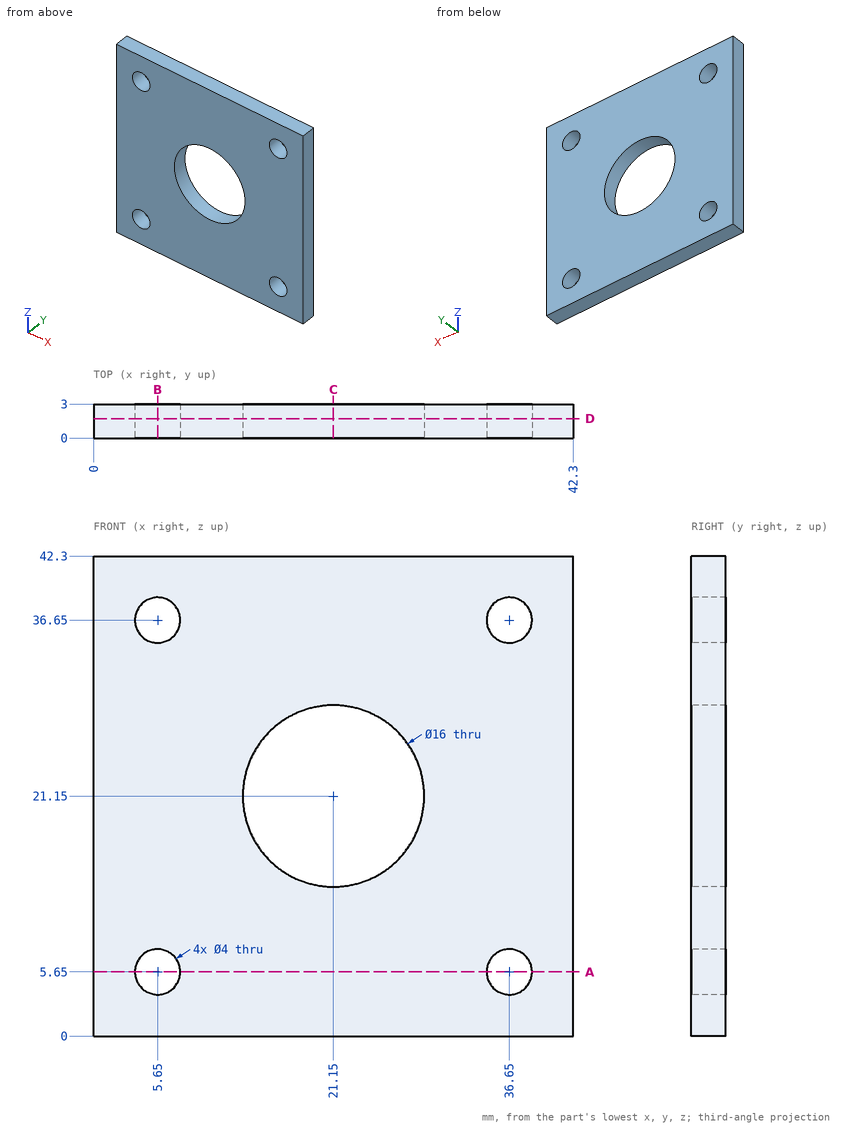
Answer from the drawing. Dimensions are ordinates in mm from the lowest x, y and z of the part. Give positions to 0.01 mm unless a question says otherwise; leave off trailing zeros. Order: outer loops, then holes, each group sorted by start corner. A loop starts at its lowest first (then second) coordinate and runs counter-clockwise, first axis right, second up. Notation, with made-up numbers: (-1.75, 15.25) - (26.25, 15.25) arc R34 ccw to (26.25, 51.25) - close; hole circle Ø8 at (-32, 58.25). An arc over 180 degrees is marked (long way). One line per item, written item: value. Start each with the question number.
1. Section B-B, the plane x = 5.65 is taken. Write down the section's boundary in (y, z).
2. Section C-C, the plane x = 21.15 is taken. Write down the section's boundary in (y, z).
3. Consider line 1 (Z direction, x = 5.65, y = 2.35); line 2 (Z direction, x = 21.15, y = 1.7). Determine where each line is inside the solid, lowest interval first.
4. This flat-tipped pin is pushed along its axis until it touches: pin 1 Ø3 at (x, z) = (5.65, 5.65) entering from -Y. Where does it stop, or does it pass through?
5. Section D-D, the plane y = 1.7 is taken. Write down the section's boundary in (x, z), then the cut area to 3 significant figures.
6. Section A-A, the plane z = 5.65 is taken. Write down the section's boundary in (x, y), then the cut area to 3 significant figures.
Filled sheet:
1. outline: (0, 0) - (3, 0) - (3, 3.65) - (0, 3.65) - close; (0, 7.65) - (3, 7.65) - (3, 34.65) - (0, 34.65) - close; (0, 38.65) - (3, 38.65) - (3, 42.3) - (0, 42.3) - close
2. outline: (0, 0) - (3, 0) - (3, 13.15) - (0, 13.15) - close; (0, 29.15) - (3, 29.15) - (3, 42.3) - (0, 42.3) - close
3. line 1: 0 to 3.65, 7.65 to 34.65, 38.65 to 42.3
3. line 2: 0 to 13.15, 29.15 to 42.3
4. pin 1: through
5. outline: (0, 0) - (42.3, 0) - (42.3, 42.3) - (0, 42.3) - close; hole circle Ø4 at (5.65, 5.65); hole circle Ø4 at (5.65, 36.65); hole circle Ø16 at (21.15, 21.15); hole circle Ø4 at (36.65, 5.65); hole circle Ø4 at (36.65, 36.65)
5. area: 1,540 mm²
6. outline: (0, 0) - (3.65, 0) - (3.65, 3) - (0, 3) - close; (7.65, 0) - (34.65, 0) - (34.65, 3) - (7.65, 3) - close; (38.65, 0) - (42.3, 0) - (42.3, 3) - (38.65, 3) - close
6. area: 103 mm²
